For this review, take the finished solid that the model builds, in its own axes (mm). Round coordinates to 2 decimals unless told otherwise and drop trailing zeros. Order: outer loops, then holes, each group sorted by start corner. A loop starts at its lowest first (then second) coordinate and runs counter-clockwise, first axis right, second up.
```python
from build123d import *

# Parameters (mm, degrees)
EXTRUDE_1_DEPTH = 2500


with BuildPart() as part:
    # Model → Бобышка-Вытянуть1 (new body)
    with BuildSketch(Plane.XY):
        with BuildLine():
            Line((-11.5, -10), (-10.5, -11))
            Line((-10.5, -11), (10.5, -11))
            Line((10.5, -11), (11.5, -10))
            Line((11.5, -10), (11.5, -5))
            Line((11.5, -5), (8.5, -3))
            Line((8.5, -3), (8.5, 2))
            Line((8.5, 2), (9.007584586, 2.507584586))
            ThreePointArc((9.007584586, 2.507584586), (9.732233047, 4.080761184), (11.305409645, 4.805409645))
            Line((11.305409645, 4.805409645), (11.5, 5))
            Line((11.5, 5), (11.5, 8))
            Line((11.5, 8), (11.305409645, 8.194590355))
            ThreePointArc((11.305409645, 8.194590355), (9.732233047, 8.919238816), (9.007584586, 10.492415414))
            Line((9.007584586, 10.492415414), (8.5, 11))
            Line((8.5, 11), (-8.5, 11))
            Line((-8.5, 11), (-9.007584586, 10.492415414))
            ThreePointArc((-9.007584586, 10.492415414), (-9.732233047, 8.919238816), (-11.305409645, 8.194590355))
            Line((-11.305409645, 8.194590355), (-11.5, 8))
            Line((-11.5, 8), (-11.5, 5))
            Line((-11.5, 5), (-11.305409645, 4.805409645))
            ThreePointArc((-11.305409645, 4.805409645), (-9.732233047, 4.080761184), (-9.007584586, 2.507584586))
            Line((-9.007584586, 2.507584586), (-8.5, 2))
            Line((-8.5, 2), (-8.5, -3))
            Line((-8.5, -3), (-11.5, -5))
            Line((-11.5, -5), (-11.5, -10))
        make_face()
    extrude(amount=-EXTRUDE_1_DEPTH)


solid = part.part
```
Q1. Clearance check with flat-ended pins moving along their axes: pin 1 (4 mm diameter, centred on y = -1.5, z = -1651, fed in from -X); pin 2 (4 mm diameter, centred on y = -0.5, z = -710, fed in from +X). State where each tip first meets the part, or that it passes through.
Q2. Take a section at A-A, the plane z = -2059. State the section outline as (x, y) points.
Q3. Wall thickness on line 1 (X direction, y = -2, z = -1218); line 2 (X direction, y = 2.75, z = -488); line 3 (Y direction, x = -9.5, z = -2157): over which ranges is each line inside the solid? List them lowest first.
Working result:
1. pin 1: stops at x = -9.25
1. pin 2: stops at x = 8.5
2. outline: (-11.5, -10) - (-10.5, -11) - (10.5, -11) - (11.5, -10) - (11.5, -5) - (8.5, -3) - (8.5, 2) - (9.01, 2.51) arc R2.5 cw to (11.31, 4.81) - (11.5, 5) - (11.5, 8) - (11.31, 8.19) arc R2.5 cw to (9.01, 10.49) - (8.5, 11) - (-8.5, 11) - (-9.01, 10.49) arc R2.5 cw to (-11.31, 8.19) - (-11.5, 8) - (-11.5, 5) - (-11.31, 4.81) arc R2.5 cw to (-9.01, 2.51) - (-8.5, 2) - (-8.5, -3) - (-11.5, -5) - close
3. line 1: x = -8.5 to 8.5
3. line 2: x = -9.04 to 9.04
3. line 3: y = -11 to -3.67, 3.81 to 9.19
